Job drawing, mm, ordinate dimensions from the low corner. One solid piece. A direction names the side the tool comes from. Give positions to 0.01 mm unless a question says otherwise; leave off trailing zeros. Order: outer loops, then holes, each group sorted by start corner. A loop starts at its lowest first (then second) coordinate and runs counter-clockwise, first axis right, second up. Notation, with made-up numbers: M 27.25,14 L 66.25,14 A28 ccw 66.25,51 Z; hole C 19.25,34.5 d3. An arc over 180 degrees is marked long. Put each result on its own line as item: value. Start each with the question number.
1) Pin check, flat tips, straight feed: pin 1 (5 mm diameter, centred on x = 81.5, z = 7, fed in from +Y); pin 2 (4 mm diameter, centred on x = 55, z = 5, fed in from +Y); pin 3 (5 mm diameter, centred on y = 16.5, z = 6.5, fed in from -X). Stop position of each tip, or through.
2) Cut at D-D (z = 1). Write the cut outline in (x, y).
3) Cut at B-B (y = 8.5). Write the cut outline in (x, z).
4) Cut at A-A (x = 77.5). Write the cut outline in (y, z).
5) Cut at C-C (z = 5). Write the cut outline in (x, y).
6) Tool access for the marked faces 1, 2 and 3: list every direction of +Z, -Z, +X, -X, +Y, -Y with a clear straight run to the whole face (end or side of a thin tool).
7) Drill centre lines: line 1 (X direction, y = 21.5, z = 9.25); line 2 (Z direction, x = 7.5, y = 0.4); line 3 (X direction, y = 30.5, z = 6.75). Where is each one in solid material? Low to high. Write a range as [from, to].
8) Two-plate mould, pull along X, no slides. Class the marked faces 4, 5, 6 and 7: released by +X, released by -X, zero draft, split by the parting line, or undercut.
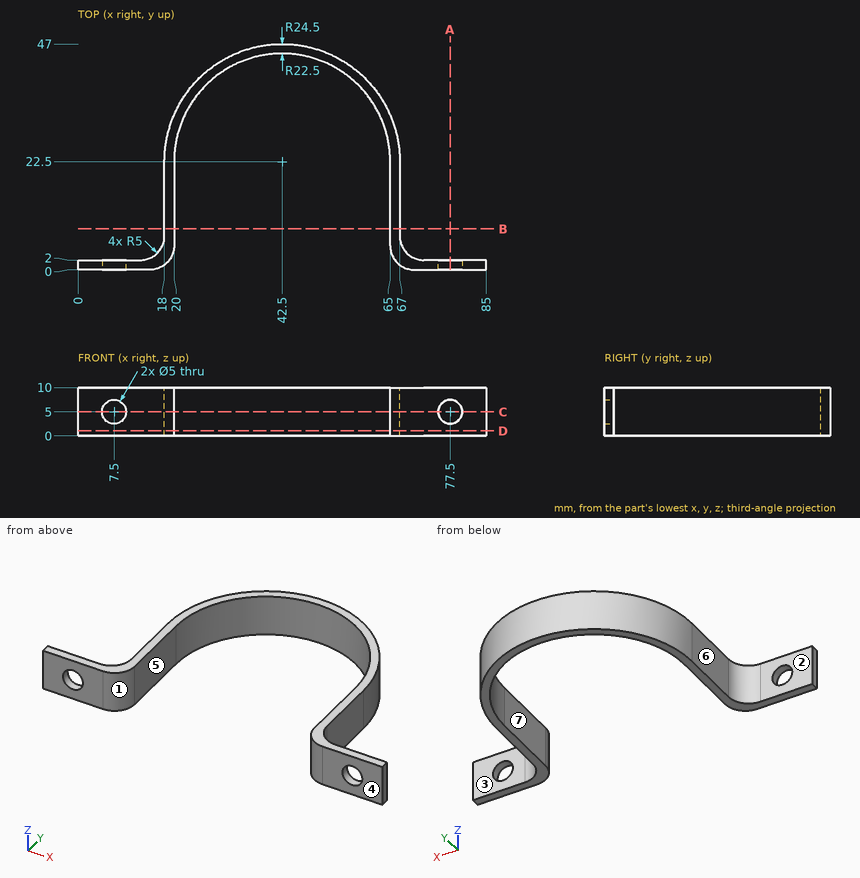
Solution:
1. pin 1: y = 2
1. pin 2: y = 44.64
1. pin 3: x = 18
2. outline: M 0,0 L 15,0 A5 ccw 20,5 L 20,22.5 A22.5 cw 65,22.5 L 65,5 A5 ccw 70,0 L 85,0 L 85,2 L 72,2 A5 cw 67,7 L 67,22.5 A24.5 ccw 18,22.5 L 18,7 A5 cw 13,2 L 0,2 Z
3. outline: M 18,0 L 20,0 L 20,10 L 18,10 Z; M 65,0 L 67,0 L 67,10 L 65,10 Z
4. outline: M 0,0 L 2,0 L 2,2.5 L 0,2.5 Z; M 0,7.5 L 2,7.5 L 2,10 L 0,10 Z
5. outline: M 0,0 L 5,0 L 5,2 L 0,2 Z; M 10,0 L 15,0 A5 ccw 20,5 L 20,22.5 A22.5 cw 65,22.5 L 65,5 A5 ccw 70,0 L 75,0 L 75,2 L 72,2 A5 cw 67,7 L 67,22.5 A24.5 ccw 18,22.5 L 18,7 A5 cw 13,2 L 10,2 Z; M 80,0 L 85,0 L 85,2 L 80,2 Z
6. face 1: +Z, -Z, -Y
6. face 2: +Z, -Z, -X, +Y
6. face 3: +Z, -Z, +X, +Y
7. line 1: [18, 20], [65, 67]
7. line 2: [0, 2.5], [7.5, 10]
7. line 3: [19.34, 21.47], [63.53, 65.66]
8. face 4: zero draft
8. face 5: undercut
8. face 6: released by -X
8. face 7: undercut
